Part model, mm, in its own coordinate system. Face numbers are marked on the shaded views. A direction names the side the tool comes from. Round coordinates to 2 decimals unless told otherwise and drop trailing zeros. Loops run counter-clockwise (first coordinate to the right, second up) from the corner with the lowest first, then second, coordinate; pieces in that order, holes last. Notation, with made-up numbers: (24, 60.5) -> (43, 60.5) arc R23 ccw to (43, 85.5) -> close; hole circle Ø9 at (23.5, -28.5). An arc over 180 degrees is marked (long way). Answer as CSV lines item,"result".
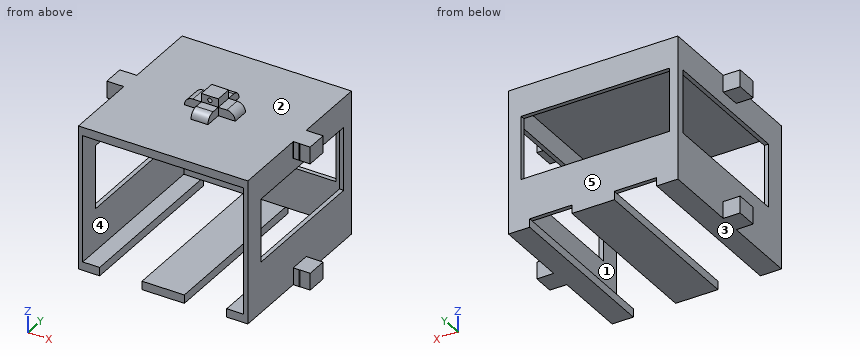
Autodesk Inventor part; units mm, degrees
ref_plane "YZ Plane" through (0, 0, 0) normal (1, 0, 0) x (0, 1, 0)
ref_plane "XZ Plane" through (0, 0, 0) normal (0, 1, 0) x (-1, 0, 0)
ref_plane "XY Plane" through (0, 0, 0) normal (0, 0, 1) x (1, 0, 0)
sketch "Esboço1" plane through (0, 0, 0) normal (0, 0, 1) x (1, 0, 0)
  line L0 (0, 0) -> (40, 0)
  line L1 (40, 0) -> (40, 40)
  line L2 (40, 40) -> (0, 40)
  line L3 (0, 40) -> (0, 0)
  dimension "d0" = 40
  dimension "d1" = 40
extrude "Extrusão1" add sketch "Esboço1" along normal blind 2
sketch "Esboço2" plane through (0, 0, 2) normal (0, 0, 1) x (1, 0, 0)
  line L0 (0, 40) -> (0, 0)
  line L1 (0, 0) -> (1, 0)
  line L2 (0, 0) -> (40, 0)
  line L3 (0, 0) -> (0, 40)
  line L4 (40, 40) -> (0, 40)
  line L5 (40, 0) -> (40, 40)
  line L6 (40, 40) -> (40, 0)
  line L7 (40, 0) -> (39, 0)
  line L8 (39, 0) -> (39, 39)
  line L9 (39, 39) -> (1, 39)
  line L10 (1, 39) -> (1, 0)
extrude "Extrusão2" add sketch "Esboço2" along normal blind 10 contours L4 L5 L2 L8 L9 L10 L1 L0
sketch "Esboço3" plane through (0, 0, 12) normal (0, 0, 1) x (1, 0, 0)
  line L0 (0, 40) -> (2, 40)
  line L1 (40, 40) -> (0, 40)
  line L2 (1, 39) -> (39, 39)
  line L3 (2, 39) -> (1, 39)
  line L4 (1, 39) -> (1, 38)
  line L5 (1, 0) -> (1, 39)
  line L6 (0, 38) -> (0, 40)
  line L7 (2, 40) -> (2, 39)
  line L8 (1, 38) -> (0, 38)
  line L9 (0, 40) -> (0, 0)
extrude "Extrusão3" add sketch "Esboço3" along normal blind 20
sketch "Esboço4" plane through (0, 0, 12) normal (0, 0, 1) x (1, 0, 0)
  line L0 (40, 40) -> (37, 40)
  line L1 (40, 40) -> (0, 40)
  line L2 (39, 39) -> (1, 39)
  line L3 (37, 39) -> (39, 39)
  line L4 (39, 39) -> (39, 37)
  line L5 (39, 39) -> (39, 0)
  line L6 (40, 0) -> (40, 40)
  line L7 (40, 37) -> (40, 40)
  line L8 (37, 40) -> (37, 39)
  line L9 (39, 37) -> (40, 37)
  line L10 (40, 40) -> (37, 40)
  line L11 (37, 39) -> (39, 39)
  line L12 (39, 39) -> (39, 37)
  point P0 (0, 0)
extrude "Extrusão4" add sketch "Esboço4" along normal blind 20
sketch "Esboço6" plane through (0, 0, 12) normal (0, 0, 1) x (1, 0, 0)
  line L0 (0, 38) -> (0, 0)
  line L1 (1, 0) -> (1, 38)
  line L2 (0, 0) -> (1, 0)
  line L3 (1, 0) -> (1, 5)
  line L4 (1, 5) -> (0, 5)
  line L5 (0, 5) -> (0, 0)
  line L6 (0, 0) -> (40, 0)
  line L7 (39, 0) -> (39, 39)
  line L8 (40, 0) -> (39, 0)
  line L9 (39, 0) -> (39, 5)
  line L10 (39, 5) -> (40, 5)
  line L11 (40, 5) -> (40, 0)
extrude "Extrusão5" add sketch "Esboço6" along normal blind 20
sketch "Esboço7" plane through (0, 0, 32) normal (0, 0, 1) x (1, 0, 0)
  line L0 (0, 38) -> (0, 5)
  line L1 (0, 38) -> (1, 38)
  line L2 (1, 5) -> (1, 38)
  line L3 (1, 38) -> (1, 5)
  line L4 (1, 5) -> (0, 5)
  line L5 (0, 40) -> (0, 38)
  line L6 (0, 5) -> (0, 38)
  point P0 (0, 0)
extrude "Extrusão6" add sketch "Esboço7" against normal blind 5
sketch "Esboço8" plane through (0, 0, 32) normal (0, 0, 1) x (1, 0, 0)
  line L0 (2, 40) -> (0, 40)
  line L1 (39, 39) -> (1, 39)
  line L2 (2, 40) -> (37, 40)
  line L3 (37, 40) -> (37, 39)
  line L4 (37, 39) -> (2, 39)
  line L5 (2, 39) -> (2, 40)
  point P0 (0, 0)
extrude "Extrusão7" add sketch "Esboço8" against normal blind 5
sketch "Esboço9" plane through (0, 0, 32) normal (0, 0, 1) x (1, 0, 0)
  line L0 (40, 0) -> (40, 40)
  line L1 (39, 37) -> (40, 37)
  line L2 (40, 37) -> (40, 5)
  line L3 (40, 5) -> (39, 5)
  line L4 (39, 5) -> (39, 37)
  point P0 (0, 0)
extrude "Extrusão8" add sketch "Esboço9" against normal blind 5
sketch "Esboço10" plane through (0, 0, 32) normal (0, 0, 1) x (1, 0, 0)
  line L0 (40, 40) -> (0, 40)
  line L1 (0, 40) -> (0, 0)
  line L2 (40, 40) -> (0, 40)
  line L3 (0, 40) -> (0, 0)
  line L4 (0, 0) -> (40, 0)
  line L5 (40, 0) -> (40, 40)
extrude "Extrusão9" add sketch "Esboço10" along normal blind 2
sketch "Esboço14" plane through (0, 0, 34) normal (0, 0, 1) x (1, 0, 0)
  line L0 (0, 40) -> (0, 0)
  line L1 (0, 40) -> (0, 20)
  circle A0 centre (-1.4378, 20) radius 2.5
  line L2 (-1.4378, 17.5) -> (-0.8668, 18) construction
  line L3 (-0.8668, 18) -> (0, 17.5) construction
  spline S0 degree 2 poles (-1.4378, 17.5) (-0.8668, 18) (0, 17.5) knots 1 1 1 2 2 2
  line L4 (40, 0) -> (40, 40)
  line L5 (40, 40) -> (40, 0)
  line L6 (40, 40) -> (0, 40)
  line L7 (0, 40) -> (0, 0)
  circle A1 centre (41.4279, 20) radius 2.5
  line L8 (41.4279, 17.5) -> (40.8569, 18) construction
  line L9 (40.8569, 18) -> (39.9901, 17.5) construction
  spline S1 degree 2 poles (41.4279, 17.5) (40.8569, 18) (39.9901, 17.5) knots 1 1 1 2 2 2
  line L10 (-1.4378, 20) -> (40, 20)
  line L11 (-1.4378, 22.5) -> (-0.8668, 22) construction
  line L12 (-0.8668, 22) -> (0, 22.5) construction
  spline S2 degree 2 poles (-1.4378, 22.5) (-0.8668, 22) (0, 22.5) knots 1 1 1 2 2 2
  spline S3 degree 2 poles (41.4279, 22.5) (40.8569, 22) (39.9901, 22.5) knots 1 1 1 2 2 2
  line L13 (41.4279, 22.5) -> (40.8569, 22) construction
  line L14 (40.8569, 22) -> (39.9901, 22.5) construction
  point P0 (40, 22.4943)
  point P1 (40, 17.5057)
  point P2 (0, 22.5)
  dimension "d30" = 5
extrude "Extrusão11" add sketch "Esboço14" against normal blind 4 contours L0 A0 S2 | L0 A0 S0 S2 | S3 A1 L4 | A1 S3 S1 L4 | L0 S0 A0 | A1 S1 L4
sketch "Esboço15" plane through (0, 0, 0) normal (0, 0, -1) x (-1, 0, 0)
  spline S0 degree 2 poles (1.4304, 17.5) (0.8594, 18) (-0.0074, 17.5) knots 1 1 1 2 2 2
  line L0 (1.4304, 17.5) -> (0.8594, 18) construction
  line L1 (0.8594, 18) -> (-0.0074, 17.5) construction
  circle A0 centre (1.4304, 20) radius 2.5
  spline S1 degree 2 poles (1.4304, 22.5) (0.8594, 22) (-0.0074, 22.5) knots 1 1 1 2 2 2
  line L2 (1.4304, 22.5) -> (0.8594, 22) construction
  line L3 (0.8594, 22) -> (-0.0074, 22.5) construction
  line L4 (-40, 40) -> (0, 40)
  line L5 (-40, 40) -> (-40, 0)
  line L6 (-39, 0) -> (-39, 39)
  spline S2 degree 2 poles (-41.4206, 17.5) (-40.8496, 18) (-39.9828, 17.5) knots 1 1 1 2 2 2
  line L7 (-41.4206, 17.5) -> (-40.8496, 18) construction
  line L8 (-40.8496, 18) -> (-39.9828, 17.5) construction
  circle A1 centre (-41.4206, 20) radius 2.5
  spline S3 degree 2 poles (-41.4206, 22.5) (-40.8496, 22) (-39.9828, 22.5) knots 1 1 1 2 2 2
  line L9 (-41.4206, 22.5) -> (-40.8496, 22) construction
  line L10 (-40.8496, 22) -> (-39.9828, 22.5) construction
  line L11 (0, 40) -> (0, 0)
  line L12 (0, 17.9497) -> (0, 22.0503)
  line L13 (-40, 0) -> (-40, 40)
  line L14 (-40, 17.9428) -> (-40, 22.0572)
  line L15 (-40, 17.9428) -> (-40, 22.0572)
  line L16 (-0.0074, 17.5) -> (3.9926, 17.5)
  line L17 (3.9926, 17.5) -> (3.9926, 22.5)
  line L18 (3.9926, 22.5) -> (-0.0074, 22.5)
  line L19 (-0.0074, 22.5) -> (-0.0074, 17.5)
  point P0 (1.4378, 22.5)
  point P1 (0, 17.5043)
  point P2 (0, 22.4957)
  point P3 (-40, 17.5099)
  point P4 (-40, 22.4901)
  dimension "d51" = 4
extrude "Extrusão12" add sketch "Esboço15" against normal blind 4 contours S0 A0 L11 S1 | L5 A1 S3 | S0 L11 A0 | L11 S1 A0 | L5 A1 S2 S3 | L5 S2 A1
sketch "Esboço20" plane through (0, 0, 2) normal (0, 0, 1) x (1, 0, 0)
  line L0 (0, 0) -> (40, 0)
  line L1 (0, 0) -> (10, 0)
  line L2 (10, 40) -> (0, 40)
  line L3 (0, 40) -> (0, 0)
  line L4 (40, 40) -> (0, 40)
  line L5 (25, 0) -> (35, 0)
  line L6 (35, 0) -> (35, 40)
  line L7 (35, 40) -> (25, 40)
  line L8 (25, 40) -> (25, 0)
  line L9 (1, 0) -> (39, 0)
  line L10 (5, 0) -> (15, 0)
  line L11 (15, 0) -> (15, 40)
  line L12 (15, 40) -> (5, 40)
  line L13 (5, 40) -> (5, 0)
  dimension "d44" = 10
  dimension "d45" = 10
  dimension "d46" = 40
extrude "Extrusão15" cut sketch "Esboço20" against normal blind 10 contours L13 L2 L4 L11 L0 | L8 L4 L6 L0
sketch "Esboço21" plane through (0, 0, 34) normal (0, 0, 1) x (1, 0, 0)
  line L0 (0, 40) -> (0, 22.5)
  line L1 (0, 22.5) -> (-4, 22.5)
  line L2 (-4, 22.5) -> (-4, 17.5)
  line L3 (-4, 17.5) -> (0, 17.5)
  line L4 (0, 17.5) -> (0, 22.5)
  point P0 (0, 0)
extrude "Extrusão16" add sketch "Esboço21" against normal blind 4
sketch "Esboço22" plane through (0, 0, 0) normal (0, 0, -1) x (-1, 0, 0)
  line L0 (0, 22.4957) -> (0, 17.5043)
  line L1 (0, 22.5) -> (4, 22.5)
  line L2 (0, 17.5043) -> (4, 17.5043)
  line L3 (4, 17.5043) -> (4, 22.5)
  line L4 (4, 22.5) -> (0, 22.5)
  line L5 (0, 22.5) -> (0, 17.5043)
  point P0 (0, 0)
extrude "Extrusão17" add sketch "Esboço22" against normal blind 4
sketch "Esboço23" plane through (0, 0, 34) normal (0, 0, 1) x (1, 0, 0)
  line L0 (40, 0) -> (40, 17.5099)
  line L1 (40, 17.5099) -> (44, 17.5099)
  line L2 (44, 17.5099) -> (44, 22.5099)
  line L3 (44, 22.5099) -> (40, 22.5099)
  line L4 (40, 22.5099) -> (40, 17.5099)
  point P0 (0, 0)
  dimension "d54" = 5
extrude "Extrusão18" add sketch "Esboço23" against normal blind 4
sketch "Esboço24" plane through (0, 0, 0) normal (0, 0, -1) x (-1, 0, 0)
  line L0 (-40, 22.4901) -> (-40, 40)
  line L1 (-41.6498, 17.5099) -> (-44, 17.5099)
  line L2 (-40, 22.5099) -> (-44, 22.5099)
  line L3 (-44, 22.5099) -> (-44, 17.5099)
  line L4 (-44, 17.5099) -> (-40, 17.5099)
  line L5 (-40, 17.5099) -> (-40, 22.5099)
  point P0 (0, 0)
  dimension "d57" = 5
extrude "Extrusão19" add sketch "Esboço24" against normal blind 4
sketch "Esboço26" plane through (0, 0, 34) normal (0, 0, 1) x (1, 0, 0)
  line L0 (0, 40) -> (0, 22.5)
  line L1 (0, 40) -> (20, 40)
  line L2 (15, 40) -> (5, 40)
  line L3 (20, 40) -> (20, 20)
  line L4 (20, 20) -> (20, 22)
  line L5 (20, 20) -> (20, 18)
  line L6 (20, 40) -> (20, 20)
  line L7 (25, 40) -> (15, 40)
  line L8 (20, 20) -> (22, 20)
  line L9 (20, 20) -> (18, 20)
  line L10 (18, 20) -> (18, 22)
  line L11 (18, 22) -> (20, 22)
  line L12 (22, 22) -> (22, 20)
  line L13 (22, 22) -> (20, 22)
  line L14 (22, 20) -> (22, 18)
  line L15 (22, 18) -> (20, 18)
  line L16 (18, 18) -> (18, 20)
  line L17 (18.1558, 18) -> (20, 18)
  line L18 (18, 18) -> (18.1677, 18)
  point P0 (0, 0)
extrude "Extrusão20" add sketch "Esboço26" along normal blind 4
sketch "Esboço27" plane through (0, 0, 34) normal (0, 0, 1) x (1, 0, 0)
  line L0 (22, 22) -> (22, 18)
  line L1 (22, 18) -> (22, 14)
  line L2 (22, 14) -> (18, 14)
  line L3 (18, 14) -> (18, 18)
  line L4 (18, 18) -> (14, 18)
  line L5 (14, 18) -> (14, 22)
  line L6 (18, 22) -> (22, 22)
  line L7 (14, 22) -> (18, 22)
  line L8 (18, 22) -> (18, 26)
  line L9 (18, 26) -> (22, 26)
  line L10 (22, 26) -> (22, 22)
  line L11 (22, 22) -> (26, 22)
  line L12 (26, 22) -> (26, 18)
  line L13 (26, 18) -> (22, 18)
  point P0 (0, 0)
extrude "Extrusão21" add sketch "Esboço27" along normal blind 2
fillet "Arredondamento1" radius 2 4 edges at (26, 20, 36) (20, 26, 36) (14, 20, 36) (20, 14, 36)
sketch "Esboço30" plane through (18, 18, 38) normal (0, -1, 0) x (1, 0, 0)
  line L0 (4, -2) -> (0, -2)
  line L1 (0, -2) -> (0, -1)
  line L2 (0, -1) -> (4, -1)
  line L3 (4, -1) -> (2, -1)
  circle A0 centre (2, -1) radius 0.5
  point P0 (-18, -38)
  dimension "d65" = 1
extrude "Extrusão22" cut sketch "Esboço30" against normal through all
properties part number "elevador_caixa_com_estabi v2"
Q1. Saw through at B-B, the plane x = 27.5. Write the cut outline in (y, z).
Geometry results:
outline,"(0, 32) -> (39, 32) -> (39, 27) -> (40, 27) -> (40, 34) -> (0, 34) -> close; (39, 2) -> (40, 2) -> (40, 12) -> (39, 12) -> close"
Q2. Two-plate mould, pull along X, no slides. Class the marked faces 4 and 5: pulls with the +X half, pulls with the -X half, needs draft (parallel to the pull), parting line crosses it, or undercut.
Geometry results:
face 4,"undercut"
face 5,"needs draft"
Q3. Saw through at A-A, the plane y = 12. Write the cut outline in (x, z).
Geometry results:
outline,"(0, 0) -> (5, 0) -> (5, 2) -> (1, 2) -> (1, 12) -> (0, 12) -> close; (0, 27) -> (1, 27) -> (1, 32) -> (39, 32) -> (39, 27) -> (40, 27) -> (40, 34) -> (0, 34) -> close; (15, 0) -> (25, 0) -> (25, 2) -> (15, 2) -> close; (35, 0) -> (40, 0) -> (40, 12) -> (39, 12) -> (39, 2) -> (35, 2) -> close"
Q4. Which spindle directions (+Z, -Z, +X, -X, +Y, -Y) get a long thin tool onto all of the face, cutting with end or side? Do the marked faces 1, 2 and 3. Say none if no direction does.
Geometry results:
face 1,"-Y"
face 2,"+Z"
face 3,"-Z, +X, -X, +Y, -Y"
Q5. Drill centre lines: line 1 along Z through (x, y) = (20, 19); line 2 along X through (y, z) = (20.35, 37); line 3 along Y through (x, z) = (39.5, 18). Where is each one in solid material? Low to high.
Geometry results:
line 1,"0 to 2, 32 to 36.5, 37.5 to 38"
line 2,"18 to 19.5, 20.5 to 22"
line 3,"0 to 5, 37 to 40"
Q6. Saw through at C-C, the plane z = 6. Write the cut outline in (x, y), then the cut area to 3 significant figures.
Geometry results:
outline,"(0, 0) -> (1, 0) -> (1, 39) -> (39, 39) -> (39, 0) -> (40, 0) -> (40, 40) -> (0, 40) -> close"
area,"118 mm2"
Q7. Drop flat-ended pins along their axis: P1, Ø0.6, axis at x = 19.5, z = 37.5, coming from the +Y side; P2, Ø1.6, axis at y = 16, z = 1, coming from the +X side; P3, Ø0.6, axis at x = 23.5, z = 35.5, coming from the -Y side. Give the stop position or say it passes through.
Geometry results:
P1,"y = 22"
P2,"x = 40"
P3,"y = 18"
Q8. Saw through at D-D, the plane x = 17. Write the cut outline in (y, z).
Geometry results:
outline,"(0, 0) -> (40, 0) -> (40, 12) -> (39, 12) -> (39, 2) -> (0, 2) -> close; (0, 32) -> (39, 32) -> (39, 27) -> (40, 27) -> (40, 34) -> (22, 34) -> (22, 36) -> (18, 36) -> (18, 34) -> (0, 34) -> close"
